Can you work these out from the drawing? Everything is in mm from the part's minimum corner. A direction names the side the tool comes from. Coordinates: 2 decimals unless noted, no trailing zeros. Loops run counter-clockwise (first coordinate to the right, second up) from the corner with the lowest first, then second, coordinate; pieces in that order, holes last. Notation, with made-up numbers: M -17,86.25 L 27,86.25 A18 cw 27,106.25 Z; hole C -16.75,28.5 d3. An arc over 180 degrees is marked long. Write each question's results on one line, items separated by ' | '.
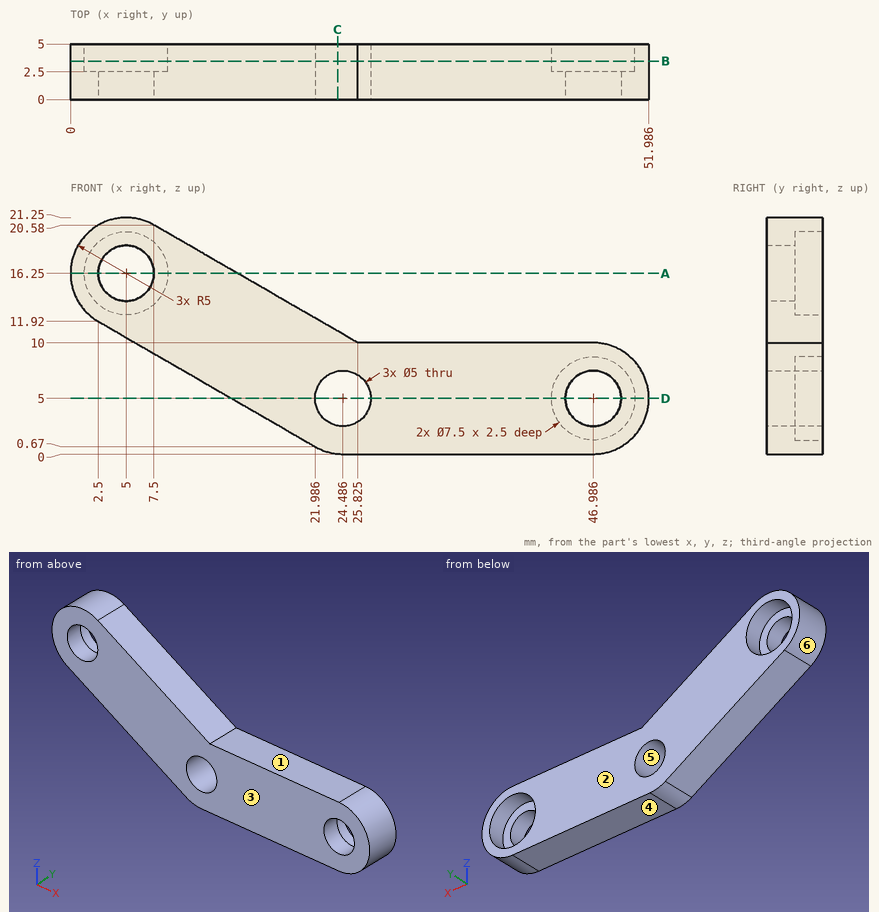
(1) Which directions (+Z, -Z, +X, -X, +Y, -Y) give clear straight access to the entire face, cutting with the end or side of a thin tool? Please do the marked faces 1 and 2.
Reported:
face 1: +Z, +X, +Y, -Y | face 2: +Z, -Z, +X, -X, +Y
(2) Will these pins go through, and if not, where does the flat tip stop? P1, Ø7, axis at x = 5, z = 16.25, coming from the +Y side; P2, Ø1.5, axis at x = 41.5, y = 2, coming from the +Z side; P3, Ø3, axis at x = 5, z = 16.25, coming from the -Y side.
Reported:
P1: stops at y = 2.5 | P2: stops at z = 10 | P3: passes through
(3) Please list where these lines run through material, in increasing order: probe 1 along X at (y, z) = (3.15, 5) (1 decimal); probe 2 along Z at (x, y) = (29, 2.45); probe 3 along X at (y, z) = (3.75, 1.75) (1 decimal). Write a range as from..to.
Reported:
probe 1: x = 14.5..22, 27..43.2, 50.7..52 | probe 2: z = 0..10 | probe 3: x = 20.1..45.1, 48.9..50.8
(4) Imagine slicing it at B-B, the plane y = 3.45. State how many separate pieces and enclosed holes the cut face has.
Reported:
separate pieces: 1 | enclosed holes: 3
(5) Imagine slicing it at C-C, the plane x = 24. List the corners of the cut face in (y, z) for me.
Reported:
outline: M 0,0.02 L 5,0.02 L 5,2.55 L 0,2.55 Z; M 0,7.45 L 5,7.45 L 5,11.05 L 0,11.05 Z
(6) Imagine slicing it at A-A, the plane z = 16.25. List the corners of the cut face in (x, y) for me.
Reported:
outline: M 0,0 L 2.5,0 L 2.5,2.5 L 1.25,2.5 L 1.25,5 L 0,5 Z; M 7.5,0 L 15,0 L 15,5 L 8.75,5 L 8.75,2.5 L 7.5,2.5 Z
(7) Imagine slicing it at D-D, the plane z = 5. List the corners of the cut face in (x, y) for me (1 decimal).
Reported:
outline: M 14.5,0 L 22,0 L 22,5 L 14.5,5 Z; M 27,0 L 44.5,0 L 44.5,2.5 L 43.2,2.5 L 43.2,5 L 27,5 Z; M 49.5,0 L 52,0 L 52,5 L 50.7,5 L 50.7,2.5 L 49.5,2.5 Z
(8) If we mould it in two halves opening along Z, with no side actions, what happens to the marked faces 3, 4, 5 and 6? For each: released by +Z, released by -Z, zero draft, split by the parting line, or undercut.
Reported:
face 3: zero draft | face 4: released by -Z | face 5: undercut | face 6: split by the parting line
